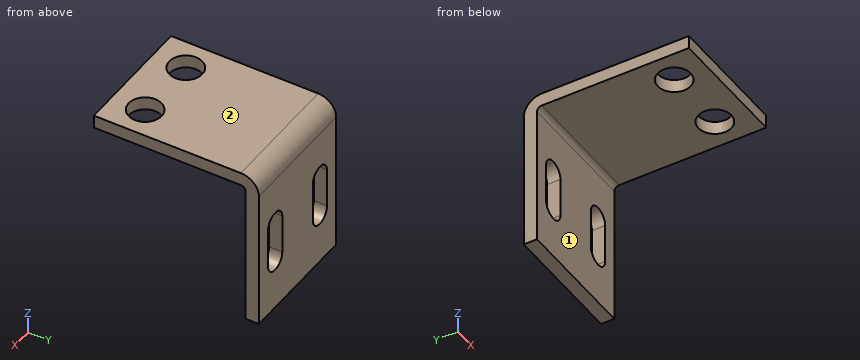
```python
from build123d import *

# Parameters (mm, degrees)
SKETCH_1_W                       = 19
SKETCH_1_H                       = 25
SKETCH_1_R                       = 2.5
SM_BASE_FLANGE_1_DEPTH           = 2
SM_EDGE_FLANGE_1_STRIP_W         = 9.4732
SM_EDGE_FLANGE_1_STRIP_H         = 2
SM_EDGE_FLANGE_1_STRIP_CUT_DEPTH = 19
SM_EDGE_FLANGE_1_DEPTH           = 19
CUT_EXTRUDE_1_DEPTH              = 10


# Sheet-metal steps are written as plain solids
with BuildPart() as part:
    # Sketch 1 → 基体-法兰1 (new body)
    with BuildSketch(Plane.XY):
        Rectangle(SKETCH_1_W, SKETCH_1_H)
        with Locations((-5, -7.5)):
            Circle(SKETCH_1_R, mode=Mode.SUBTRACT)
        with Locations((5, -7.5)):
            Circle(SKETCH_1_R, mode=Mode.SUBTRACT)
    extrude(amount=-SM_BASE_FLANGE_1_DEPTH)

    # 边线-法兰1 strip (across the edge) → 边线-法兰1 strip cut (cut)
    with BuildSketch(Plane(origin=(-9.5, 12.5, -2), x_dir=(0, -1, 0), z_dir=(1, 0, 0))):
        with Locations((-2, -1)):
            Rectangle(SM_EDGE_FLANGE_1_STRIP_W, SM_EDGE_FLANGE_1_STRIP_H)
    extrude(amount=SM_EDGE_FLANGE_1_STRIP_CUT_DEPTH, mode=Mode.SUBTRACT)

    # 边线-法兰1 section (across the edge) → 边线-法兰1 (add)
    with BuildSketch(Plane(origin=(-9.5, 12.5, -2), x_dir=(0, -1, 0), z_dir=(1, 0, 0))):
        with BuildLine():
            Line((0, 0.7366), (0, 22))
            Line((0, 22), (2, 22))
            Line((2, 22), (2, 0.7366))
            ThreePointArc((2, 0.7366), (2.215745145, 0.215745145), (2.7366, 0))
            Line((2.7366, 0), (2.7366, -2))
            ThreePointArc((2.7366, -2), (0.801531583, -1.198468417), (0, 0.7366))
        make_face()
    extrude(amount=SM_EDGE_FLANGE_1_DEPTH)

    # 草图6 → 切除-拉伸1 (cut)
    with BuildSketch(Plane(origin=(0, 12.5, 0), x_dir=(1, 0, 0), z_dir=(0, 1, 0))):
        with BuildLine():
            Line((-7.25, 10), (-7.25, 16))
            ThreePointArc((-7.25, 16), (-5.5, 17.75), (-3.75, 16))
            Line((-3.75, 16), (-3.75, 10))
            ThreePointArc((-3.75, 10), (-5.5, 8.25), (-7.25, 10))
        make_face()
        with BuildLine():
            Line((3.75, 10), (3.75, 16))
            ThreePointArc((3.75, 16), (5.5, 17.75), (7.25, 16))
            Line((7.25, 16), (7.25, 10))
            ThreePointArc((7.25, 10), (5.5, 8.25), (3.75, 10))
        make_face()
    extrude(amount=-CUT_EXTRUDE_1_DEPTH, mode=Mode.SUBTRACT)


solid = part.part
```
Source: CAD feature listing. Evaluate the final solid. Frame: model axes, mm. Face numbers are marked on the shaded views. A direction names the side the tool comes from. Round coordinates to 2 decimals unless told otherwise and drop trailing zeros. Loops run counter-clockwise (first coordinate to the right, second up) from the corner with the lowest first, then second, coordinate; pieces in that order, holes last. Notation, with made-up numbers: M 38,-24 L 44,-24 A16 ccw 44,3 Z; hole C 52.25,-35.75 d10. An arc over 180 degrees is marked long. Put each result on its own line as item: value.
(1) Section C-C, the plane x = 4.5. Return loops of the section in (y, z), and give its area (3 significant figures).
Solutions:
outline: M -12.5,-2 L -9.95,-2 L -9.95,0 L -12.5,0 Z; M -5.05,-2 L 9.76,-2 A0.74 cw 10.5,-2.74 L 10.5,-8.56 L 12.5,-8.56 L 12.5,-2.74 A2.74 ccw 9.76,0 L -5.05,0 Z; M 10.5,-24 L 12.5,-24 L 12.5,-17.44 L 10.5,-17.44 Z
area: 65.0 mm²
(2) First-contact query: pin 1 (1 mm diameter, centred on x = -3, z = -5, fed in from -Y); pin 2 (10 mm diameter, centred on x = -2.5, y = -3, fed in from -Z); pin 3 (3 mm diameter, centred on x = -5, y = -7.5, fed in from +Z). Flat tips, straight axial feed; report the tip coordinate or a pass-through.
Solutions:
pin 1: y = 10.5
pin 2: z = -2
pin 3: through
(3) Section A-A, the plane y = -5.5. Return loops of the section in (x, z), and give its area (3 significant figures).
Solutions:
outline: M -9.5,-2 L -6.5,-2 L -6.5,0 L -9.5,0 Z; M -3.5,-2 L 3.5,-2 L 3.5,0 L -3.5,0 Z; M 6.5,-2 L 9.5,-2 L 9.5,0 L 6.5,0 Z
area: 26.0 mm²
(4) Section D-D, the plane x = -0.75. Return loops of the section in (y, z).
Solutions:
outline: M -12.5,-2 L 9.76,-2 A0.74 cw 10.5,-2.74 L 10.5,-24 L 12.5,-24 L 12.5,-2.74 A2.74 ccw 9.76,0 L -12.5,0 Z
(5) Ray query, line 1 (Y direction, x = -1, z = -17.75); line 2 (Z direction, x = 0, y = 3.5); line 3 (Y direction, x = 5, z = -1.4). Return the intervals inside material, ascending. Write a range as [from, to].
Solutions:
line 1: [10.5, 12.5]
line 2: [-2, 0]
line 3: [-12.5, -10], [-5, 12.15]
(6) Section B-B, the plane z = -11.5. Return loops of the section in (x, y).
Solutions:
outline: M -9.5,10.5 L -7.25,10.5 L -7.25,12.5 L -9.5,12.5 Z; M -3.75,10.5 L 3.75,10.5 L 3.75,12.5 L -3.75,12.5 Z; M 7.25,10.5 L 9.5,10.5 L 9.5,12.5 L 7.25,12.5 Z
(7) Access query for the marked faces 1 and 2. Directions: +Z, -Z, +X, -X, +Y, -Y. A direction counts if a zero-diameter tool reaches every point of the face in a straight line with its end or side. Return the directions, or none.
Solutions:
face 1: -Z, +X, -X, -Y
face 2: +Z, +X, -X, +Y, -Y
